```python
from build123d import *

# Parameters (mm, degrees)
SKETCH1_R                = 10
BOSS_EXTRUDE1_DEPTH      = 200
BOSS_EXTRUDE2_DEPTH      = 15
BOSS_EXTRUDE2_DEPTH_BACK = 15
SKETCH2_W                = 125
SKETCH2_H                = 20
BOSS_EXTRUDE3_DEPTH      = 10
BOSS_EXTRUDE3_DEPTH_BACK = 10
SKETCH3_W                = 25
SKETCH3_H                = 75


with BuildPart() as part:
    # Sketch1 → Boss-Extrude1 (new body)
    with BuildSketch(Plane(origin=(0, 0, 0), x_dir=(1, 0, 0), z_dir=(0, 1, 0))):
        with Locations(Location((0, 0, 0), (0, 0, 270))):
            Circle(SKETCH1_R)
    extrude(amount=BOSS_EXTRUDE1_DEPTH)

    # Sketch2 → Boss-Extrude2 (add, two sides: drawn at the far end of the back side and taken through both)
    with BuildSketch(Plane(origin=(0, 0, 0), x_dir=(0, 0, -1), z_dir=(1, 0, 0)).offset(-BOSS_EXTRUDE2_DEPTH_BACK)):
        with Locations((0, 210)):
            Rectangle(SKETCH2_W, SKETCH2_H)
    extrude(amount=BOSS_EXTRUDE2_DEPTH + BOSS_EXTRUDE2_DEPTH_BACK)

    # Sketch3 → Boss-Extrude3 (add, two sides: drawn at the far end of the back side and taken through both)
    with BuildSketch(Plane(origin=(0, 0, 0), x_dir=(0, 0, -1), z_dir=(1, 0, 0)).offset(-BOSS_EXTRUDE3_DEPTH_BACK)):
        with Locations((-50, 257.5)):
            Rectangle(SKETCH3_W, SKETCH3_H)
        with Locations((50, 257.5)):
            Rectangle(SKETCH3_W, SKETCH3_H)
    extrude(amount=BOSS_EXTRUDE3_DEPTH + BOSS_EXTRUDE3_DEPTH_BACK)


solid = part.part
```
Geometry check sheet. Reference: the model listing, model coordinates, mm. A direction names the side the tool comes from. Give positions to 0.01 mm unless a question says otherwise; leave off trailing zeros. Write each loop counter-clockwise with the first axis right and the second up, starting at its lowest first coordinate (ties: lowest second). Pieces come first, ordered by that corner, then holes.
1) Access from +Z, -Z, +X, -X, +Y, -Y to the whole of each face (thin tool, end or side, straight path). Record for faces 1 (the flat face through (0, 295, -50)), 2 (the flat face through (-10, 258, -50)), 3 (the flat face through (10, 258, 50)), 4 (the cylindrical face through (-9.76, 98.6, -2.17)), 5 (the flat face through (0, 257, -37.5)).
2) Section check C-C, the plane x = 0. Record the boundary of the cut face in (y, z), and give its area (4 significant figures).
3) Gauge pin test, flat ends, axial feed: pin 1 (20 mm diameter, centred on y = 270, z = -52, fed in from -X); pin 2 (2 mm diameter, centred on x = 8, y = 165, fed in from +Z); pin 3 (4 mm diameter, centred on x = -1, y = 129, fed in from -Z); pin 4 (2 mm diameter, centred on y = 254, z = -35.5, fed in from +X). Record the tip position at first contact, or that the pin passes through.
4) Release check for a two-part mould opening along Z. For faces 6 (the flat face through (10, 258, -50)), 7 (the flat face through (0, 257, 37.5)), 8 (the flat face through (0, 247, -62.5)) record: pulls with the +Z half, pulls with the -Z half, needs draft (parallel to the pull), parting line crosses it, or undercut.
5) Section check D-D, the plane z = 26. Record the boundary of the cut face in (x, y), and give its area (3 significant figures).
6) Section check A-A, the plane y = 236.5. Record the boundary of the cut face in (x, z).
7) Material ranges on L1, parallel to Z at x = 8.5, y = 234; L2, parallel to Y at x = 6, z = 50; L3, parallel to Y at x = -10.75, z = -11, recorded low to high.
8) Section check B-B, the plane z = 0. Record the boundary of the cut face in (x, y), and give its area (3 significant figures).
Computed:
1. face 1: +Z, -Z, +X, -X, +Y
1. face 2: +Z, -Z, -X, +Y
1. face 3: +Z, -Z, +X, +Y
1. face 4: -Y
1. face 5: +X, -X, +Y
2. outline: (0, -10) - (200, -10) - (200, -62.5) - (295, -62.5) - (295, -37.5) - (220, -37.5) - (220, 37.5) - (295, 37.5) - (295, 62.5) - (200, 62.5) - (200, 10) - (0, 10) - close
2. area: 10,250 mm2
3. pin 1: stops at x = -10
3. pin 2: stops at z = 7.14
3. pin 3: stops at z = -10
3. pin 4: passes through
4. face 6: needs draft
4. face 7: undercut
4. face 8: pulls with the -Z half
5. outline: (-15, 200) - (15, 200) - (15, 220) - (-15, 220) - close
5. area: 600 mm2
6. outline: (-10, -62.5) - (10, -62.5) - (10, -37.5) - (-10, -37.5) - close; (-10, 37.5) - (10, 37.5) - (10, 62.5) - (-10, 62.5) - close
7. L1: z = -62.5 to -37.5, 37.5 to 62.5
7. L2: y = 200 to 295
7. L3: y = 200 to 220
8. outline: (-15, 200) - (-10, 200) - (-10, 0) - (10, 0) - (10, 200) - (15, 200) - (15, 220) - (-15, 220) - close
8. area: 4,600 mm2
